Build history of the part. All positions in model axes, mm. Face numbers are marked on the shaded views. A direction names the side the tool comes from. Coordinates: 2 decimals unless noted, no trailing zeros. Write each loop counter-clockwise with the first axis right and the second up, starting at its lowest first coordinate (ties: lowest second). Pieces come first, ordered by that corner, then holes. Notation, with made-up numbers: (21.5, 12.25) -> (40.5, 12.25) arc R10 cw to (40.5, 28.25) -> close; hole circle Ø6 at (7, 65.25). An arc over 180 degrees is marked (long way). Write each question's results on one line, items separated by ' | '. Start each with the question number.
Q1. Two-plate mould, pull along X, no slides. Class the marked faces 4, 5, 6 and 7: released by +X, released by -X, zero draft, split by the parting line, or undercut.
Q2. Tool access for the marked faces 1, 2 and 3: list every direction of +Z, -Z, +X, -X, +Y, -Y with a clear straight run to the whole face (end or side of a thin tool).
Q3. Drop flat-ended pins along their axis: pin 1 Ø5 at (x, z) = (-13, -43.5) entering from +Y; pin 2 Ø16 at (x, z) = (-18, -33.5) entering from -Y. Give the stop position or say it passes through.
Q4. Saw through at B-B on x = -19.05. Give the cut face in (y, z) (3 decimals).
Q5. Saw through at C-C on z = -25.4. Give the cut face in (x, y).
Q6. Drill centre lines: line 1 (X direction, y = 9.5, z = -41); line 2 (Z direction, x = -17, y = -22.5) (3 decimals); line 3 (Y direction, x = -19.05, z = -49.6). Where is each one in solid material? Low to high.
Q7. Saw through at D-D on y = 12.7. Give the cut face in (x, z).
Autodesk Inventor part; units mm, degrees
ref_plane "YZ Plane" through (0, 0, 0) normal (1, 0, 0) x (0, 1, 0)
ref_plane "XZ Plane" through (0, 0, 0) normal (0, 1, 0) x (-1, 0, 0)
ref_plane "XY Plane" through (0, 0, 0) normal (0, 0, 1) x (1, 0, 0)
sketch "Sketch1" plane through (0, 0, 0) normal (0, 1, 0) x (-1, 0, 0)
  line L0 (0, 0) -> (38.1, 0)
  line L1 (38.1, 0) -> (38.1, -50.8)
  line L2 (38.1, -50.8) -> (0, -50.8)
  line L3 (0, -50.8) -> (0, 0)
  line L4 (38.1, -50.8) -> (33.02, -50.8)
  line L5 (33.02, -50.8) -> (33.02, 0)
  line L6 (33.02, 0) -> (38.1, 0)
  line L7 (38.1, 0) -> (38.1, -50.8)
  line L8 (0, -50.8) -> (5.08, -50.8)
  line L9 (5.08, -50.8) -> (5.08, 0)
  line L10 (5.08, 0) -> (0, 0)
  line L11 (0, 0) -> (0, -50.8)
  dimension "d0" = 38.1
  dimension "d1" = 50.8
  dimension "d2" = 5.08
  dimension "d3" = 5.08
extrude "Extrusion1" add sketch "Sketch1" along normal blind 25.4 contours L0 L9 L2 L3 | L0 L1 L2 L5
extrude "Extrusion2" add sketch "Sketch1" against normal blind 5.08
sketch "Sketch2" plane through (0, 25.4, 0) normal (1, 0, 0) x (0, 0, -1)
  line L0 (50.8, 0) -> (0, 0)
  line L1 (25.4, 0) -> (25.4, -12.7)
  point P0 (0, -25.4)
  dimension "d8" = 12.7
hole "Hole1" at (0, 12.7, -25.4) direction (-1, 0, 0) diameter 6.7564 end through all
sketch "Sketch3" plane through (0, -5.08, 0) normal (0, -1, 0) x (1, 0, 0)
  line L0 (0, -50.8) -> (-5.08, -50.8)
  line L1 (0, -50.8) -> (0, -38.1)
  line L2 (0, 0) -> (0, -50.8)
  line L3 (0, -38.1) -> (0, -12.7)
  line L4 (0, -38.1) -> (-19.05, -38.1)
  line L5 (0, -12.7) -> (-19.05, -12.7)
  line L6 (-38.1, -50.8) -> (-38.1, 0)
  line L7 (0, -39.6875) -> (-38.1, -39.6875)
  line L8 (-38.1, -39.6875) -> (-38.1, -36.5125)
  line L9 (-38.1, -36.5125) -> (0, -36.5125)
  line L10 (0, -36.5125) -> (0, -39.6875)
  line L11 (0, -39.6875) -> (-38.1, -36.5125) construction
  line L12 (-38.1, -39.6875) -> (0, -36.5125) construction
  line L13 (0, -11.1125) -> (-38.1, -11.1125)
  line L14 (-38.1, -11.1125) -> (-38.1, -14.2875)
  line L15 (-38.1, -14.2875) -> (0, -14.2875)
  line L16 (0, -14.2875) -> (0, -11.1125)
  line L17 (0, -11.1125) -> (-38.1, -14.2875) construction
  line L18 (-38.1, -11.1125) -> (0, -14.2875) construction
  line L19 (-38.1, 0) -> (-38.1, -50.8)
  line L20 (-38.1, 0) -> (0, 0)
  line L21 (0, 0) -> (0, -3.175)
  line L22 (0, -3.175) -> (-38.1, -3.175)
  line L23 (-38.1, -3.175) -> (-38.1, 0)
  line L24 (0, -50.8) -> (-38.1, -50.8)
  line L25 (-38.1, -50.8) -> (-38.1, -47.625)
  line L26 (-38.1, -47.625) -> (0, -47.625)
  line L27 (0, -47.625) -> (0, -50.8)
  dimension "d16" = 12.7
  dimension "d17" = 25.4
  dimension "d18" = 19.05
  dimension "d19" = 3.175
  dimension "d20" = 3.175
  dimension "d32" = 3.175
  dimension "d33" = 3.175
extrude "Extrusion3" add sketch "Sketch3" along normal blind 25.4 contours L0 L24 L6 L26 L1 | L6 L20 L2 L22
sketch "Sketch4" plane through (-38.1, -5.08, 0) normal (0, 0, 1) x (1, 0, 0)
  line L0 (38.1, -25.4) -> (19.05, -25.4)
  line L1 (19.05, -25.4) -> (19.05, -13.97)
  point P0 (38.1, 5.08)
  dimension "d23" = 11.43
hole "Hole2" at (-19.05, -19.05, 0) direction (0, 0, -1) diameter 2.8575 end through all
fillet "Fillet1" radius 3.175 6 edges at (-38.1, -2.54, 0) (0, -2.54, 0) (0, -2.54, -50.8) (-38.1, -2.54, -50.8) (0, -5.08, -25.4) (-38.1, -5.08, -25.4)
properties part number "Sample Holder end for 8020-thruhole-widestance"
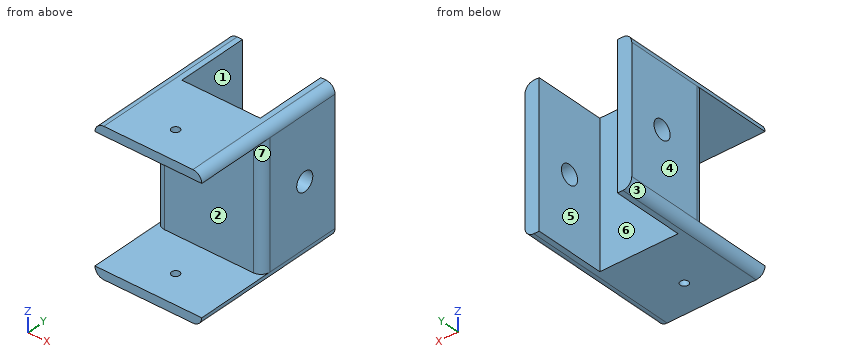
Returned:
1) face 4: released by -X | face 5: undercut | face 6: undercut | face 7: released by +X
2) face 1: +Z, -Z, +Y | face 2: +X, -X, -Y | face 3: -Z, -X, +Y, -Y
3) pin 1: stops at y = 0 | pin 2: stops at y = -5.08
4) outline: (-30.48, -50.8) -> (-20.479, -50.8) -> (-20.479, -47.625) -> (-30.48, -47.625) -> close; (-30.48, -3.175) -> (-20.479, -3.175) -> (-20.479, 0) -> (-30.48, 0) -> close; (-17.621, -50.8) -> (0, -50.8) -> (0, 0) -> (-17.621, 0) -> (-17.621, -3.175) -> (-5.08, -3.175) -> (-5.08, -47.625) -> (-17.621, -47.625) -> close
5) outline: (-38.1, -1.91) arc R3.17 ccw to (-34.93, -5.08) -> (-3.17, -5.08) arc R3.17 ccw to (0, -1.91) -> (0, 9.32) -> (-5.08, 9.32) -> (-5.08, 0) -> (-33.02, 0) -> (-33.02, 9.32) -> (-38.1, 9.32) -> close; (-38.1, 16.08) -> (-33.02, 16.08) -> (-33.02, 25.4) -> (-38.1, 25.4) -> close; (-5.08, 16.08) -> (0, 16.08) -> (0, 25.4) -> (-5.08, 25.4) -> close
6) line 1: x = -38.1 to -33.02, -5.08 to 0 | line 2: z = -50.8 to -47.625, -3.175 to 0 | line 3: y = -30.48 to -20.48, -17.62 to 0
7) outline: (-38.1, -47.63) arc R3.17 ccw to (-34.93, -50.8) -> (-33.02, -50.8) -> (-33.02, -28.78) -> (-38.1, -28.78) -> close; (-38.1, -22.02) -> (-33.02, -22.02) -> (-33.02, 0) -> (-34.93, 0) arc R3.17 ccw to (-38.1, -3.17) -> close; (-5.08, -50.8) -> (-3.17, -50.8) arc R3.17 ccw to (0, -47.63) -> (0, -28.78) -> (-5.08, -28.78) -> close; (-5.08, -22.02) -> (0, -22.02) -> (0, -3.17) arc R3.17 ccw to (-3.17, 0) -> (-5.08, 0) -> close
